```python
from build123d import *

# Parameters (mm, degrees)
SKETCH1_W           = 112.776
SKETCH1_H           = 96.774
BOSS_EXTRUDE1_DEPTH = 12.7
CUT_EXTRUDE2_START  = -12.7
SKETCH2_R           = 8.334375
CUT_EXTRUDE2_DEPTH  = 25.4
CUT_EXTRUDE4_START  = -12.7
SKETCH3_R           = 8.334375
CUT_EXTRUDE4_DEPTH  = 25.4
CUT_EXTRUDE6_START  = -12.7
SKETCH4_R           = 11.509375
CUT_EXTRUDE6_DEPTH  = 12.7
CUT_EXTRUDE8_START  = -12.7
SKETCH5_R           = 11.509375
CUT_EXTRUDE8_DEPTH  = 12.7
CUT_EXTRUDE10_START = 12.7
SKETCH6_R           = 11.509375
CUT_EXTRUDE10_DEPTH = 12.7
CUT_EXTRUDE12_START = 12.7
SKETCH7_R           = 11.509375
CUT_EXTRUDE12_DEPTH = 12.7
CUT_EXTRUDE14_START = 12.7
SKETCH8_R           = 16.6497
CUT_EXTRUDE14_DEPTH = 2.8194
CUT_EXTRUDE16_START = 12.7
SKETCH9_R           = 16.6497
CUT_EXTRUDE16_DEPTH = 2.8194
CUT_EXTRUDE18_START = -12.7
SKETCH10_R          = 3.571875
CUT_EXTRUDE18_DEPTH = 7.874
CUT_EXTRUDE20_START = -12.7
SKETCH11_R          = 3.571875
CUT_EXTRUDE20_DEPTH = 7.874
CUT_EXTRUDE22_START = 12.7
SKETCH12_R          = 3.175
CUT_EXTRUDE22_DEPTH = 7.874
CUT_EXTRUDE24_START = 12.7
SKETCH13_R          = 3.175
CUT_EXTRUDE24_DEPTH = 7.874


with BuildPart() as part:
    # Sketch1 → Boss-Extrude1 (new, symmetric)
    with BuildSketch(Plane(origin=(0, 0, 0), x_dir=(0, 1, 0), z_dir=(0, 0, 1))):
        Rectangle(SKETCH1_W, SKETCH1_H)
    extrude(amount=BOSS_EXTRUDE1_DEPTH, both=True)

    # Sketch2 → Cut-Extrude2 (cut)
    with BuildSketch(Plane(origin=(0, 0, 0), x_dir=(0, 1, 0), z_dir=(0, 0, 1)).offset(CUT_EXTRUDE2_START)):
        with Locations(Location((-40.513, -32.512, 0), (0, 0, 90))):
            Circle(SKETCH2_R)
    extrude(amount=CUT_EXTRUDE2_DEPTH, mode=Mode.SUBTRACT)

    # Sketch3 → Cut-Extrude4 (cut)
    with BuildSketch(Plane(origin=(0, 0, 0), x_dir=(0, 1, 0), z_dir=(0, 0, 1)).offset(CUT_EXTRUDE4_START)):
        with Locations(Location((40.513, -32.512, 0), (0, 0, 90))):
            Circle(SKETCH3_R)
        with Locations(Location((-40.513, 32.512, 0), (0, 0, 90))):
            Circle(SKETCH3_R)
        with Locations(Location((40.513, 32.512, 0), (0, 0, 90))):
            Circle(SKETCH3_R)
    extrude(amount=CUT_EXTRUDE4_DEPTH, mode=Mode.SUBTRACT)

    # Sketch4 → Cut-Extrude6 (cut)
    with BuildSketch(Plane(origin=(0, 0, 0), x_dir=(0, 1, 0), z_dir=(0, 0, 1)).offset(CUT_EXTRUDE6_START)):
        with Locations(Location((-27.813, 0, 0), (0, 0, 270))):
            Circle(SKETCH4_R)
    extrude(amount=CUT_EXTRUDE6_DEPTH, mode=Mode.SUBTRACT)

    # Sketch5 → Cut-Extrude8 (cut)
    with BuildSketch(Plane(origin=(0, 0, 0), x_dir=(0, 1, 0), z_dir=(0, 0, 1)).offset(CUT_EXTRUDE8_START)):
        with Locations(Location((18.161, 0, 0), (0, 0, 270))):
            Circle(SKETCH5_R)
    extrude(amount=CUT_EXTRUDE8_DEPTH, mode=Mode.SUBTRACT)

    # Sketch6 → Cut-Extrude10 (cut)
    with BuildSketch(Plane(origin=(0, 0, 0), x_dir=(0, 1, 0), z_dir=(0, 0, 1)).offset(CUT_EXTRUDE10_START)):
        with Locations(Location((-18.161, 0, 0), (0, 0, 270))):
            Circle(SKETCH6_R)
    extrude(amount=-CUT_EXTRUDE10_DEPTH, mode=Mode.SUBTRACT)

    # Sketch7 → Cut-Extrude12 (cut)
    with BuildSketch(Plane(origin=(0, 0, 0), x_dir=(0, 1, 0), z_dir=(0, 0, 1)).offset(CUT_EXTRUDE12_START)):
        with Locations(Location((27.813, 0, 0), (0, 0, 270))):
            Circle(SKETCH7_R)
    extrude(amount=-CUT_EXTRUDE12_DEPTH, mode=Mode.SUBTRACT)

    # Sketch8 → Cut-Extrude14 (cut)
    with BuildSketch(Plane(origin=(0, 0, 0), x_dir=(0, 1, 0), z_dir=(0, 0, 1)).offset(CUT_EXTRUDE14_START)):
        with Locations(Location((-18.161, 0, 0), (0, 0, 270))):
            Circle(SKETCH8_R)
    extrude(amount=-CUT_EXTRUDE14_DEPTH, mode=Mode.SUBTRACT)

    # Sketch9 → Cut-Extrude16 (cut)
    with BuildSketch(Plane(origin=(0, 0, 0), x_dir=(0, 1, 0), z_dir=(0, 0, 1)).offset(CUT_EXTRUDE16_START)):
        with Locations(Location((27.813, 0, 0), (0, 0, 270))):
            Circle(SKETCH9_R)
    extrude(amount=-CUT_EXTRUDE16_DEPTH, mode=Mode.SUBTRACT)

    # Sketch10 → Cut-Extrude18 (cut)
    with BuildSketch(Plane(origin=(0, 0, 0), x_dir=(0, 1, 0), z_dir=(0, 0, 1)).offset(CUT_EXTRUDE18_START)):
        with Locations(Location((49.149, 0, 0), (0, 0, 270))):
            Circle(SKETCH10_R)
    extrude(amount=CUT_EXTRUDE18_DEPTH, mode=Mode.SUBTRACT)

    # Sketch11 → Cut-Extrude20 (cut)
    with BuildSketch(Plane(origin=(0, 0, 0), x_dir=(0, 1, 0), z_dir=(0, 0, 1)).offset(CUT_EXTRUDE20_START)):
        with Locations(Location((0.127, -32.512, 0), (0, 0, 270))):
            Circle(SKETCH11_R)
    extrude(amount=CUT_EXTRUDE20_DEPTH, mode=Mode.SUBTRACT)

    # Sketch12 → Cut-Extrude22 (cut)
    with BuildSketch(Plane(origin=(0, 0, 0), x_dir=(0, 1, 0), z_dir=(0, 0, 1)).offset(CUT_EXTRUDE22_START)):
        with Locations(Location((-49.149, 0, 0), (0, 0, 270))):
            Circle(SKETCH12_R)
    extrude(amount=-CUT_EXTRUDE22_DEPTH, mode=Mode.SUBTRACT)

    # Sketch13 → Cut-Extrude24 (cut)
    with BuildSketch(Plane(origin=(0, 0, 0), x_dir=(0, 1, 0), z_dir=(0, 0, 1)).offset(CUT_EXTRUDE24_START)):
        with Locations(Location((-0.127, 32.512, 0), (0, 0, 270))):
            Circle(SKETCH13_R)
    extrude(amount=-CUT_EXTRUDE24_DEPTH, mode=Mode.SUBTRACT)


solid = part.part
```
Here's how the part is built. I have some questions about the finished solid (model axes, mm). A direction names the side the tool comes from. Round coordinates to 2 decimals unless told otherwise and drop trailing zeros. Write each loop counter-clockwise with the first axis right and the second up, starting at its lowest first coordinate (ties: lowest second). Pieces come first, ordered by that corner, then holes. Notation, with made-up numbers: M 61.5,60.25 L 66.5,60.25 A21 cw 66.5,74.25 Z; hole C -26.75,65.25 d9. An arc over 180 degrees is marked long. Answer as CSV lines item,"result". Start each with the question number.
1. On a 3-axis mill with a long thin cutter (end or side, diameter ignored), from which of +Z, -Z, +X, -X, +Y, -Y can I reach the whole of each face in a straight line? I mean faces 1 (the flat face through (0, -33, 0)), 2 (the flat face through (-1, -1, -12.7)), 3 (the flat face through (0, 31, 0)). Say none if no direction works.
2. Suppose I cut it at D-D on z = 8.25. Count the separate pieces of the cut face and the enclosed holes in it, then the cut area to 3 significant figures.
3. Thinking about a two-plate mould opening in X: for faces 4 (the flat face through (-1, -1, 12.7)), 5 (the cylindrical face through (-13.21, 17.68, 11.31)), 6 (the flat face through (32, 0, -4.826)), which applies, released by +X, released by -X, zero draft, split by the parting line, or undercut?
4. I need wall thicknesses on probe 1 along Y at (x, z) = (0, 11.1); probe 2 along Y at (x, z) = (0, 2.5); probe 3 along Y at (x, z) = (6, 5). Which ranges of each line are inside material? Lowest first, please.
5. Suppose I cut it at C-C on x = 6.5. Write out the boundary of the cut face in (y, z), then the cut area to 3 significant figures.
6. Suppose I cut it at A-A on y = 26. Write out the boundary of the cut face in (x, z), then the cut area to 3 significant figures.
7. Suppose I cut it at B-B on z = -1.25. Write out the boundary of the cut face in (x, y).
8. I'm going to push flat-ended pins straight in: pin 1 Ø5 at (x, y) = (5.5, -31.5) entering from -Z; pin 2 Ø3.5 at (x, y) = (-1, 48) entering from -Z; pin 3 Ø10 at (x, y) = (6.5, 32) entering from +Z; pin 4 Ø18.5 at (x, y) = (0, -18.161) entering from -Z. Where does each tip first touch, or does it pass through?
Check result:
1,face 1,"-Z"
1,face 2,"-Z, +X, -X, +Y, -Y"
1,face 3,"+Z"
2,separate pieces,"1"
2,enclosed holes,"8"
2,area,"9,150 mm2"
3,face 4,"zero draft"
3,face 5,"undercut"
3,face 6,"undercut"
4,probe 1,"y = -56.39 to -52.32, -45.97 to -34.81, -1.51 to 11.16, 44.46 to 56.39"
4,probe 2,"y = -56.39 to -29.67, -6.65 to 16.3, 39.32 to 56.39"
4,probe 3,"y = -56.39 to -27.98, -8.34 to 17.99, 37.63 to 56.39"
5,outline,"M -56.39,-12.7 L -37.31,-12.7 L -37.31,0 L -27.66,0 L -27.66,9.88 L -33.49,9.88 L -33.49,12.7 L -56.39,12.7 Z; M -18.31,-12.7 L 8.66,-12.7 L 8.66,0 L 18.31,0 L 18.31,9.88 L 12.48,9.88 L 12.48,12.7 L -2.83,12.7 L -2.83,9.88 L -8.66,9.88 L -8.66,0 L -18.31,0 Z; M 27.66,-12.7 L 56.39,-12.7 L 56.39,12.7 L 43.14,12.7 L 43.14,9.88 L 37.31,9.88 L 37.31,0 L 27.66,0 Z"
5,area,"1,830 mm2"
6,outline,"M -48.39,-12.7 L -8.43,-12.7 L -8.43,0 L -11.37,0 L -11.37,9.88 L -16.55,9.88 L -16.55,12.7 L -48.39,12.7 Z; M 8.43,-12.7 L 48.39,-12.7 L 48.39,12.7 L 16.55,12.7 L 16.55,9.88 L 11.37,9.88 L 11.37,0 L 8.43,0 Z"
6,area,"1,930 mm2"
7,outline,"M -48.39,-56.39 L 48.39,-56.39 L 48.39,56.39 L -48.39,56.39 Z; hole C -32.51,-40.51 d16.67; hole C -32.51,40.51 d16.67; hole C 0,-27.81 d23.02; hole C 0,18.16 d23.02; hole C 32.51,-40.51 d16.67; hole C 32.51,40.51 d16.67"
8,pin 1,"stops at z = 0"
8,pin 2,"stops at z = -4.83"
8,pin 3,"stops at z = 9.88"
8,pin 4,"stops at z = -12.7"
